```python
from build123d import *

# Parameters (mm, degrees)
SKETCH_1_W                       = 380
SKETCH_1_H                       = 100
EXTRUDE_1_DEPTH                  = 5
FILLET_2_R                       = 5
SKETCH_2_R                       = 1.6
CUT_EXTRUDE_1_DEPTH              = 197.53244007
PATTERN_LINEAR_1_COUNT           = 2
PATTERN_LINEAR_1_PITCH           = 20
MIRROR_1_COPY_1_SKETCH_R         = 1.6
MIRROR_1_COPY_1_DEPTH            = 197.53244007
MIRROR_2_COPY_1_SKETCH_R         = 1.6
MIRROR_2_COPY_1_DEPTH            = 197.53244007
MIRROR_2_COPY_2_SKETCH_R         = 1.6
MIRROR_2_COPY_2_DEPTH            = 197.53244007
MIRROR_2_COPY_3_SKETCH_R         = 1.6
MIRROR_2_COPY_3_DEPTH            = 197.53244007
SKETCH_3_R                       = 2.1
CUT_EXTRUDE_2_DEPTH              = 197.53244007
PATTERN_LINEAR_2_COUNT           = 3
PATTERN_LINEAR_2_PITCH           = 40
MIRROR_3_COPY_1_SKETCH_R         = 2.1
MIRROR_3_COPY_1_DEPTH            = 197.53244007
MIRROR_3_COPY_2_SKETCH_R         = 2.1
MIRROR_3_COPY_2_DEPTH            = 197.53244007
SKETCH_4_R                       = 2.1
CUT_EXTRUDE_3_DEPTH              = 197.53244007
PATTERN_LINEAR_3_COUNT           = 2
PATTERN_LINEAR_3_PITCH           = 133
PATTERN_LINEAR_3_COPY_1_SKETCH_R = 2.1
PATTERN_LINEAR_3_COPY_1_DEPTH    = 197.53244007
PATTERN_LINEAR_4_COUNT           = 2
PATTERN_LINEAR_4_PITCH           = 80
MIRROR_5_COPY_1_SKETCH_R         = 2.1
MIRROR_5_COPY_1_DEPTH            = 197.53244007
MIRROR_5_COPY_2_SKETCH_R         = 2.1
MIRROR_5_COPY_2_DEPTH            = 197.53244007
CUT_EXTRUDE_4_DEPTH              = 197.53244007
MIRROR_7_COPY_1_DEPTH            = 197.53244007


with BuildPart() as part:
    # 草图1 → 凸台-拉伸1 (new body)
    with BuildSketch(Plane(origin=(0, 0, 0), x_dir=(1, 0, 0), z_dir=(0, 1, 0))):
        Rectangle(SKETCH_1_W, SKETCH_1_H)
    extrude(amount=EXTRUDE_1_DEPTH)

    # 圆角2
    fillet_2_edges = [part.edges().sort_by_distance(p)[0] for p in [
        (190, 2.5, 50),
        (-190, 2.5, 50),
        (-190, 2.5, -50),
        (190, 2.5, -50),
    ]]
    fillet(fillet_2_edges, radius=FILLET_2_R)

    # 草图2 → 切除-拉伸1 (cut, through all)
    with BuildSketch(Plane(origin=(0, 5, 0), x_dir=(1, 0, 0), z_dir=(0, 1, 0))):
        with Locations(Location((177, 15, 0), (0, 0, 270))):
            Circle(SKETCH_2_R)
    cut_extrude_1 = extrude(amount=-CUT_EXTRUDE_1_DEPTH, mode=Mode.SUBTRACT)

    # 阵列(线性)1: 切除-拉伸1 ×2
    with Locations(*[(-i * PATTERN_LINEAR_1_PITCH, 0, 0) for i in range(1, PATTERN_LINEAR_1_COUNT)]):
        add(cut_extrude_1, mode=Mode.SUBTRACT)

    # 镜向1: 切除-拉伸1 across plane
    add(cut_extrude_1.mirror(Plane.XY), mode=Mode.SUBTRACT)

    # 镜向1 copy 1 sketch → 镜向1 copy 1 (cut, through all)
    with BuildSketch(Plane(origin=(-20, 5, 0), x_dir=(1, 0, 0), z_dir=(0, 1, 0))):
        with Locations((177, -15)):
            Circle(MIRROR_1_COPY_1_SKETCH_R)
    extrude(amount=-MIRROR_1_COPY_1_DEPTH, mode=Mode.SUBTRACT)

    # 镜向2: 切除-拉伸1 across plane
    add(cut_extrude_1.mirror(Plane(origin=(0, 0, 0), x_dir=(0, 0, 1), z_dir=(1, 0, 0))), mode=Mode.SUBTRACT)

    # 镜向2 copy 1 sketch → 镜向2 copy 1 (cut, through all)
    with BuildSketch(Plane(origin=(20, 5, 0), x_dir=(-1, 0, 0), z_dir=(0, 1, 0))):
        with Locations((177, -15)):
            Circle(MIRROR_2_COPY_1_SKETCH_R)
    extrude(amount=-MIRROR_2_COPY_1_DEPTH, mode=Mode.SUBTRACT)

    # 镜向2 copy 2 sketch → 镜向2 copy 2 (cut, through all)
    with BuildSketch(Plane(origin=(0, 5, 0), x_dir=(-1, 0, 0), z_dir=(0, 1, 0))):
        with Locations(Location((177, 15, 0), (0, 0, 270))):
            Circle(MIRROR_2_COPY_2_SKETCH_R)
    extrude(amount=-MIRROR_2_COPY_2_DEPTH, mode=Mode.SUBTRACT)

    # 镜向2 copy 3 sketch → 镜向2 copy 3 (cut, through all)
    with BuildSketch(Plane(origin=(20, 5, 0), x_dir=(-1, 0, 0), z_dir=(0, 1, 0))):
        with Locations(Location((177, 15, 0), (0, 0, 270))):
            Circle(MIRROR_2_COPY_3_SKETCH_R)
    extrude(amount=-MIRROR_2_COPY_3_DEPTH, mode=Mode.SUBTRACT)

    # 草图3 → 切除-拉伸2 (cut, through all)
    with BuildSketch(Plane(origin=(0, 5, 0), x_dir=(1, 0, 0), z_dir=(0, 1, 0))):
        with Locations(Location((-50, 40, 0), (0, 0, 270))):
            Circle(SKETCH_3_R)
    cut_extrude_2 = extrude(amount=-CUT_EXTRUDE_2_DEPTH, mode=Mode.SUBTRACT)

    # 阵列(线性)2: 切除-拉伸2 ×3
    with Locations(*[(0, 0, i * PATTERN_LINEAR_2_PITCH) for i in range(1, PATTERN_LINEAR_2_COUNT)]):
        add(cut_extrude_2, mode=Mode.SUBTRACT)

    # 镜向3: 切除-拉伸2 across plane
    add(cut_extrude_2.mirror(Plane(origin=(0, 0, 0), x_dir=(0, 0, 1), z_dir=(1, 0, 0))), mode=Mode.SUBTRACT)

    # 镜向3 copy 1 sketch → 镜向3 copy 1 (cut, through all)
    with BuildSketch(Plane(origin=(0, 5, 40), x_dir=(-1, 0, 0), z_dir=(0, 1, 0))):
        with Locations((-50, -40)):
            Circle(MIRROR_3_COPY_1_SKETCH_R)
    extrude(amount=-MIRROR_3_COPY_1_DEPTH, mode=Mode.SUBTRACT)

    # 镜向3 copy 2 sketch → 镜向3 copy 2 (cut, through all)
    with BuildSketch(Plane(origin=(0, 5, 80), x_dir=(-1, 0, 0), z_dir=(0, 1, 0))):
        with Locations((-50, -40)):
            Circle(MIRROR_3_COPY_2_SKETCH_R)
    extrude(amount=-MIRROR_3_COPY_2_DEPTH, mode=Mode.SUBTRACT)

    # 草图4 → 切除-拉伸3 (cut, through all)
    with BuildSketch(Plane(origin=(0, 5, 0), x_dir=(1, 0, 0), z_dir=(0, 1, 0))):
        with Locations(Location((-65.5, -26.5, 0), (0, 0, 270))):
            Circle(SKETCH_4_R)
    cut_extrude_3 = extrude(amount=-CUT_EXTRUDE_3_DEPTH, mode=Mode.SUBTRACT)

    # 镜向4: 切除-拉伸3 across plane
    add(cut_extrude_3.mirror(Plane.XY), mode=Mode.SUBTRACT)

    # 阵列(线性)3: 切除-拉伸3 ×2
    with Locations(*[(i * PATTERN_LINEAR_3_PITCH, 0, 0) for i in range(1, PATTERN_LINEAR_3_COUNT)]):
        add(cut_extrude_3, mode=Mode.SUBTRACT)

    # 阵列(线性)3 copy 1 sketch → 阵列(线性)3 copy 1 (cut, through all)
    with BuildSketch(Plane(origin=(133, 5, 0), x_dir=(1, 0, 0), z_dir=(0, 1, 0))):
        with Locations((-65.5, 26.5)):
            Circle(PATTERN_LINEAR_3_COPY_1_SKETCH_R)
    extrude(amount=-PATTERN_LINEAR_3_COPY_1_DEPTH, mode=Mode.SUBTRACT)

    # 阵列(线性)4: 切除-拉伸2 ×2
    with Locations(*[(-i * PATTERN_LINEAR_4_PITCH, 0, 0) for i in range(1, PATTERN_LINEAR_4_COUNT)]):
        add(cut_extrude_2, mode=Mode.SUBTRACT)

    # 镜向5 copy 1 sketch → 镜向5 copy 1 (cut, through all)
    with BuildSketch(Plane(origin=(80, 5, 0), x_dir=(-1, 0, 0), z_dir=(0, 1, 0))):
        with Locations((-50, -40)):
            Circle(MIRROR_5_COPY_1_SKETCH_R)
    extrude(amount=-MIRROR_5_COPY_1_DEPTH, mode=Mode.SUBTRACT)

    # 镜向5 copy 2 sketch → 镜向5 copy 2 (cut, through all)
    with BuildSketch(Plane(origin=(0, 5, 0), x_dir=(-1, 0, 0), z_dir=(0, 1, 0))):
        with Locations((-50, -40)):
            Circle(MIRROR_5_COPY_2_SKETCH_R)
    extrude(amount=-MIRROR_5_COPY_2_DEPTH, mode=Mode.SUBTRACT)

    # 草图6 → 切除-拉伸4 (cut, through all)
    with BuildSketch(Plane(origin=(0, 5, 0), x_dir=(1, 0, 0), z_dir=(0, 1, 0))):
        with BuildLine():
            Line((-132.229853022, 22.110343678), (-101.2783764, 22.110343678))
            ThreePointArc((-101.2783764, 22.110343678), (-99.192992914, 20.024960192), (-101.2783764, 17.939576706))
            Line((-101.2783764, 17.939576706), (-132.229853022, 17.939576706))
            ThreePointArc((-132.229853022, 17.939576706), (-134.315236507, 20.024960192), (-132.229853022, 22.110343678))
        make_face()
    cut_extrude_4 = extrude(amount=-CUT_EXTRUDE_4_DEPTH, mode=Mode.SUBTRACT)

    # 镜向6: 切除-拉伸4 across plane
    add(cut_extrude_4.mirror(Plane.XY), mode=Mode.SUBTRACT)

    # 镜向7: 切除-拉伸4 across plane
    add(cut_extrude_4.mirror(Plane(origin=(0, 0, 0), x_dir=(0, 0, 1), z_dir=(1, 0, 0))), mode=Mode.SUBTRACT)

    # 镜向7 copy 1 sketch → 镜向7 copy 1 (cut, through all)
    with BuildSketch(Plane(origin=(0, 5, 0), x_dir=(-1, 0, 0), z_dir=(0, 1, 0))):
        with BuildLine():
            Line((-132.229853022, 22.110343678), (-101.2783764, 22.110343678))
            ThreePointArc((-101.2783764, 22.110343678), (-99.192992914, 20.024960192), (-101.2783764, 17.939576706))
            Line((-101.2783764, 17.939576706), (-132.229853022, 17.939576706))
            ThreePointArc((-132.229853022, 17.939576706), (-134.315236507, 20.024960192), (-132.229853022, 22.110343678))
        make_face()
    extrude(amount=-MIRROR_7_COPY_1_DEPTH, mode=Mode.SUBTRACT)


solid = part.part
```
Model file for the job. Use its own axes, mm. Coordinates: 2 decimals unless noted, no trailing zeros. Answer as CSV lines item,"result".
(1) Flat gauge pin, fed straight in: pin 1 (8 mm diameter, centred on x = -93, z = -39, fed in from -Y). Where does the tip first touch, or does it go through?
Geometry says:
pin 1,"stops at y = 0"
(2) Band-saw the part on A-A, the plane y = 1.9. State how many separate pieces and enclosed holes the cut face has, then the cut area to 3 significant figures.
Geometry says:
separate pieces,"1"
enclosed holes,"24"
area,"37,200 mm2"
(3) Wall check: line 1 along X through (y, z) = (3.35, 26.5); line 2 along X through (y, z) = (1.9, -0.5); line 3 along Z through (x, y) = (68, 0.8). Give the ranges that are in metal, low to high.
Geometry says:
line 1,"x = -190 to -67.6, -63.4 to 65.4, 69.6 to 190"
line 2,"x = -190 to -52.04, -47.96 to 47.96, 52.04 to 190"
line 3,"z = -50 to -28.54, -24.46 to 24.46, 28.54 to 50"
